Answer from the drawing. Dimensions are ordinates in mm from the lowest x, y and z of the part. A direction names the side the tool comes from. Coordinates: 2 decimals unless noted, no trailing zeros. Write each loop counter-clockwise with the first axis right and the second up, starting at its lowest first coordinate (ties: lowest second). Pieces come first, ordered by that corner, then holes.
(1) Straight lines are drawn through the part: line 1 along Z through (x, y) = (69, 9); line 2 along Z through (x, y) = (69, 2.4); line 3 along Y through (x, z) = (114.5, 28). For each, find the intervals that lie inside material, in ascending order.
(2) Given pin 1 (1 mm diameter, centred on y = 10.5, z = 63, fed in from -X); pin 2 (5 mm diameter, centred on x = 69, z = 38.5, fed in from +Y); pin 3 (4 mm diameter, centred on y = 2.5, z = 25.5, fed in from +X); pin 4 (9.5 mm diameter, centred on x = 69, z = 69, fed in from +Y), each flat-ended and moving along its own axis, determine where each tip first touches the part or whether it passes through.
(3) Which of the six approach directions +Z, -Z, +X, -X, +Y, -Y give full straight-line access (tool end or side, diameter ignored) to the marked faces 1 and 2?
(4) The part is cut by section A-A, the plane z = 69. Determine the outline of the cut face in (x, y), and give its area (3 significant figures).
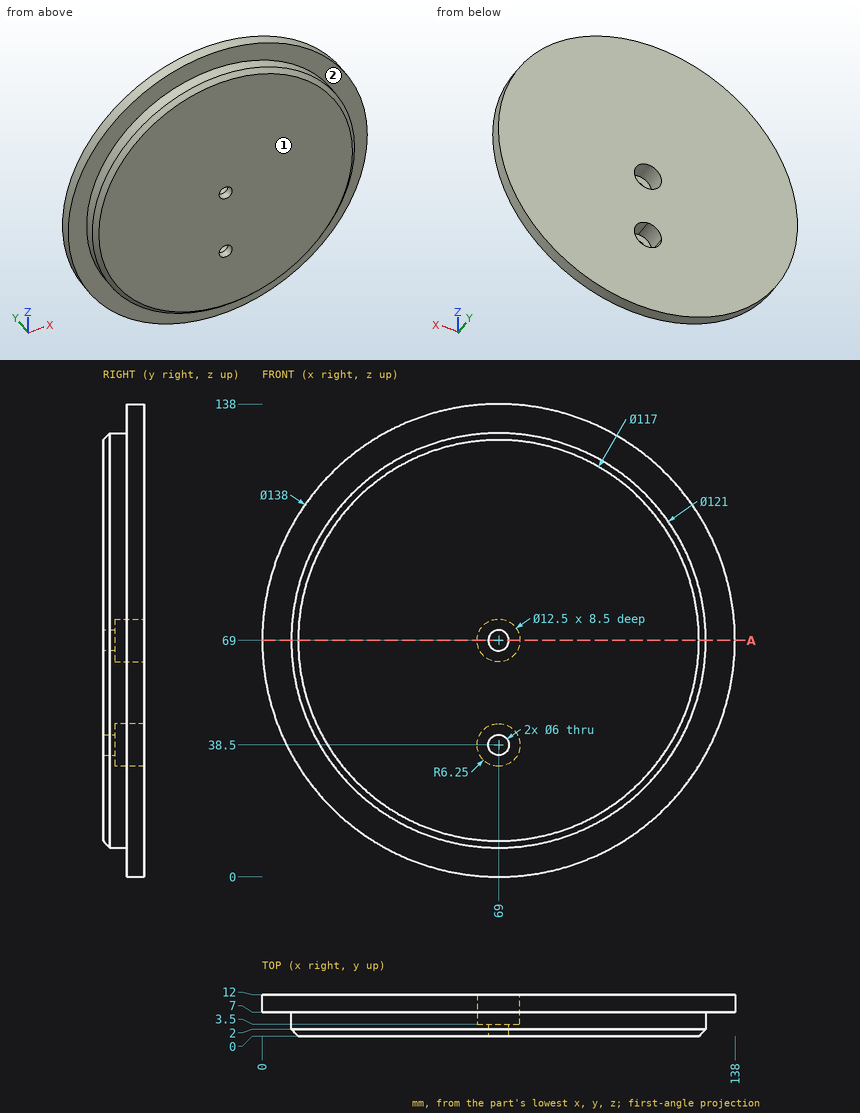
Computed:
1. line 1: z = 0 to 32.25, 44.75 to 62.75, 75.25 to 138
1. line 2: z = 8.5 to 35.5, 41.5 to 66, 72 to 129.5
1. line 3: y = 7 to 12
2. pin 1: stops at x = 0.22
2. pin 2: passes through
2. pin 3: stops at x = 113.02
2. pin 4: stops at y = 3.5
3. face 1: +Z, -Z, +X, -X, -Y
3. face 2: -Y
4. outline: (0, 7) - (8.5, 7) - (8.5, 2) - (10.5, 0) - (66, 0) - (66, 3.5) - (62.75, 3.5) - (62.75, 12) - (0, 12) - close; (72, 0) - (127.5, 0) - (129.5, 2) - (129.5, 7) - (138, 7) - (138, 12) - (75.25, 12) - (75.25, 3.5) - (72, 3.5) - close
4. area: 1,410 mm2
